```python
from build123d import *

# Parameters (mm, degrees)
F0_R      = 5
F1_DEPTH  = 3
F3_DEPTH  = 2
F6_DEPTH  = 1.3
F8_DEPTH  = 3
F10_DEPTH = 3
F12_DEPTH = 13


with BuildPart() as f1:
    # F0 (on Front) → F1 (new body)
    with BuildSketch(Plane.XZ):
        Circle(F0_R)
    extrude(amount=F1_DEPTH)

    # F2 (on Front) → F3 (join)
    with BuildSketch(Plane.XZ):
        with BuildLine():
            ThreePointArc((3.25, 2.25), (2.957107, 2.957107), (2.25, 3.25))
            Line((2.25, 3.25), (-2.25, 3.25))
            ThreePointArc((-2.25, 3.25), (-2.957107, 2.957107), (-3.25, 2.25))
            Line((-3.25, 2.25), (-3.25, -2.25))
            ThreePointArc((-3.25, -2.25), (-2.957107, -2.957107), (-2.25, -3.25))
            Line((-2.25, -3.25), (2.25, -3.25))
            ThreePointArc((2.25, -3.25), (2.957107, -2.957107), (3.25, -2.25))
            Line((3.25, -2.25), (3.25, 2.25))
        make_face()
    extrude(amount=-F3_DEPTH)

    # F5 (on face) → F6 (join)
    with BuildSketch(Plane(origin=(0, 2, 0), x_dir=(-1, 0, 0), z_dir=(0, 1, 0))):
        with BuildLine():
            Line((3.011181, 5.764368), (-3.021163, 5.764368))
            ThreePointArc((-3.021163, 5.764368), (-4.77577, 5.037585), (-5.502553, 3.282978))
            Line((-5.502553, 3.282978), (-5.502553, -5.026481))
            Line((-5.502553, -5.026481), (5.503863, -5.026481))
            Line((5.503863, -5.026481), (5.503863, 3.25))
            ThreePointArc((5.503863, 3.25), (4.781457, 5.0266), (3.011181, 5.764368))
        make_face()
    extrude(amount=F6_DEPTH)

    # F7 (on face) → F8 (join)
    with BuildSketch(Plane(origin=(0, 3.3, 0), x_dir=(-1, 0, 0), z_dir=(0, 1, 0))):
        with BuildLine():
            Line((3, 13.25), (0, 13.25))
            Line((0, 13.25), (-3, 13.25))
            ThreePointArc((-3, 13.25), (-10.071068, 10.321068), (-13, 3.25))
            Line((-13, 3.25), (-13, -12.532328))
            Line((-13, -12.532328), (0, -12.532328))
            Line((0, -12.532328), (13, -12.532328))
            Line((13, -12.532328), (13, 3.25))
            ThreePointArc((13, 3.25), (10.071068, 10.321068), (3, 13.25))
        make_face()
    extrude(amount=F8_DEPTH)

    # F9 (on face) → F10 (join)
    with BuildSketch(Plane(origin=(0, 6.3, 0), x_dir=(-1, 0, 0), z_dir=(0, 1, 0))):
        with BuildLine():
            Line((-13, 41.776921), (-13, -12.532328))
            Line((-13, -12.532328), (13, -12.532328))
            Line((13, -12.532328), (13, 41.776921))
            ThreePointArc((13, 41.776921), (11.140128, 46.267049), (6.65, 48.126921))
            Line((6.65, 48.126921), (-6.65, 48.126921))
            ThreePointArc((-6.65, 48.126921), (-11.140128, 46.267049), (-13, 41.776921))
        make_face()
    extrude(amount=F10_DEPTH)

    # F11 (on Right) → F12 (join, symmetric)
    with BuildSketch(Plane.YZ):
        with BuildLine():
            ThreePointArc((-4.499917, 44.689184), (-0.013706, 49.216576), (4.5, 44.716597))
            Line((4.5, 44.716597), (6.291118, 28.223049))
            Line((6.291118, 28.223049), (9.316304, 28.223049))
            Line((9.316304, 28.223049), (9.292265, 47.855158))
            ThreePointArc((9.292265, 47.855158), (9.263071, 48.124349), (9.177474, 48.381234))
            ThreePointArc((9.177474, 48.381234), (7.493667, 50.958381), (5.122331, 52.921456))
            ThreePointArc((5.122331, 52.921456), (2.657907, 53.992931), (0, 54.389135))
            ThreePointArc((0, 54.389135), (-9.339994, 47.231055), (-4.856021, 36.351367))
            ThreePointArc((-4.856021, 36.351367), (-4.585088, 36.351301), (-4.450556, 36.586473))
            Line((-4.450556, 36.586473), (-4.499917, 44.689184))
        make_face()
        with BuildLine():
            ThreePointArc((5.122331, 52.921456), (2.664224, 54.014979), (0, 54.389135))
            ThreePointArc((0, 54.389135), (2.657907, 53.992931), (5.122331, 52.921456))
        make_face()
    extrude(amount=F12_DEPTH, both=True)


solid = f1.part
```
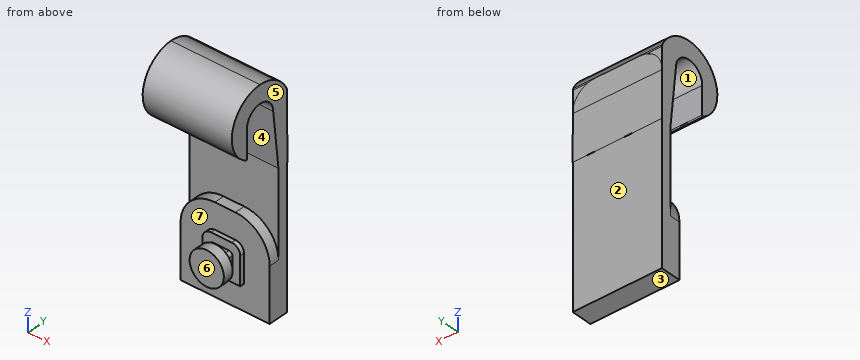
The listing builds one solid part. Answer for the finished solid, in the listing's coordinates (mm). Face numbers are marked on the shaded views. A direction names the side the tool comes from. Round coordinates to 2 decimals unless told otherwise and drop trailing zeros. Write each loop counter-clockwise with the first axis right and the second up, starting at its lowest first coordinate (ties: lowest second). Pieces come first, ordered by that corner, then holes. Notation, with made-up numbers: (59, -30.75) -> (83, -30.75) arc R24 cw to (83, -20.75) -> close; hole circle Ø9 at (83, 33). An arc over 180 degrees is marked (long way). Answer as a JSON object with one key per item and string values. Group by question number.
Q1. Each of these flat-tipped pins is pushed along its axis until it touches: pin 1 Ø12 at (x, z) = (-4, 25) entering from -Y; pin 2 Ø1.6 at (y, z) = (0.5, -0.5) entering from +X; pin 3 Ø12 at (x, z) = (2.5, 42.5) entering from +Y; pin 4 Ø5 at (x, y) = (-5.5, 1) entering from -Z. Where does it stop, or does it pass through?
Q2. Section A-A (z = 0) is taken. Write down the section's boundary in (x, y), plus the area to 3 significant figures.
Q3. Section D-D (y = -1.25) is taken. Write down the section's boundary in (x, z), plus the area to 3 significant figures.
Q4. Which of the six approach directions +Z, -Z, +X, -X, +Y, -Y give full straight-line access (tool end or side, diameter ignored) to the marked faces 5, 6 and 7?
Q5. Determine the mould class of the marked faces 1, 2, 3 and 4 for opening direction Y: pulls with the +Y half, pulls with the -Y half, needs draft (parallel to the pull), parting line crosses it, or undercut.
Q6. Straight lines are drawn through the part: line 1 along Z through (x, y) = (0.25, 8.75); line 2 along Y through (x, z) = (-7, -9); line 3 along Y through (x, z) = (-6.5, 17.5). For each, find the intervals that lie inside material, in ascending order.
Check values:
{
 "1": {"pin 1": "y = 5.99", "pin 2": "x = 5", "pin 3": "y = 9.31", "pin 4": "z = -12.53"},
 "2": {"outline": "(-13, 3.3) -> (-5.5, 3.3) -> (-5.5, 2) -> (-3.25, 2) -> (-3.25, 0) -> (-5, 0) -> (-5, -3) -> (5, -3) -> (5, 0) -> (3.25, 0) -> (3.25, 2) -> (5.5, 2) -> (5.5, 3.3) -> (13, 3.3) -> (13, 9.3) -> (-13, 9.3) -> close", "area": "213 mm^2"},
 "3": {"outline": "(-13, 49.04) -> (13, 49.04) -> (13, 54.31) -> (-13, 54.31) -> close; circle Ø10 at (0, 0)", "area": "216 mm^2"},
 "4": {"face 5": "+Z, -Z, +X, +Y, -Y", "face 6": "-Z, +X, -X, -Y", "face 7": "-Y"},
 "5": {"face 1": "undercut", "face 2": "pulls with the +Y half", "face 3": "needs draft", "face 4": "undercut"},
 "6": {"line 1": "-12.53 to 49.21", "line 2": "3.3 to 9.3", "line 3": "6.3 to 9.3"}
}
